```python
from build123d import *

# Parameters (mm, degrees)
SKETCH1_R           = 11.176
SKETCH1_R_2         = 1.5
BOSS_EXTRUDE1_DEPTH = 3.175


with BuildPart() as part:
    # Sketch1 → Boss-Extrude1 (new body)
    with BuildSketch(Plane.XY):
        with BuildLine():
            Line((-19.05, -19.05), (-19.05, 0))
            ThreePointArc((-19.05, 0), (0, 19.05), (19.05, 0))
            Line((19.05, 0), (19.05, -4.05))
            ThreePointArc((19.05, -4.05), (23.443398282, -14.656601718), (34.05, -19.05))
            Line((34.05, -19.05), (178.2, -19.05))
            ThreePointArc((178.2, -19.05), (188.806601718, -14.656601718), (193.2, -4.05))
            Line((193.2, -4.05), (193.2, 0))
            ThreePointArc((193.2, 0), (212.25, 19.05), (231.3, 0))
            Line((231.3, 0), (231.3, -19.05))
            Line((231.3, -19.05), (231.3, -79.925453532))
            Line((231.3, -79.925453532), (-19.05, -79.925453532))
            Line((-19.05, -79.925453532), (-19.05, -19.05))
        make_face()
        Circle(SKETCH1_R, mode=Mode.SUBTRACT)
        with Locations((212.25, 0)):
            Circle(SKETCH1_R, mode=Mode.SUBTRACT)
        with Locations((0, 13.9954)):
            Circle(SKETCH1_R_2, mode=Mode.SUBTRACT)
        with Locations((212.25, 13.9954)):
            Circle(SKETCH1_R_2, mode=Mode.SUBTRACT)
        with Locations((13.9954, 0)):
            Circle(SKETCH1_R_2, mode=Mode.SUBTRACT)
        with Locations((0, -13.9954)):
            Circle(SKETCH1_R_2, mode=Mode.SUBTRACT)
        with Locations((-13.9954, 0)):
            Circle(SKETCH1_R_2, mode=Mode.SUBTRACT)
        with Locations((198.2546, 0)):
            Circle(SKETCH1_R_2, mode=Mode.SUBTRACT)
        with Locations((212.25, -13.9954)):
            Circle(SKETCH1_R_2, mode=Mode.SUBTRACT)
        with Locations((226.2454, 0)):
            Circle(SKETCH1_R_2, mode=Mode.SUBTRACT)
    extrude(amount=BOSS_EXTRUDE1_DEPTH)


solid = part.part
```
Part model, mm, in its own coordinate system. A direction names the side the tool comes from. Give positions to 0.01 mm unless a question says otherwise; leave off trailing zeros. Write each loop counter-clockwise with the first axis right and the second up, starting at its lowest first coordinate (ties: lowest second). Pieces come first, ordered by that corner, then holes. Notation, with made-up numbers: (7.25, 26.5) -> (39.25, 26.5) arc R15 ccw to (39.25, 46.5) -> close; hole circle Ø10 at (26.5, -6). An arc over 180 degrees is marked (long way). Put each result on its own line as item: value. Start each with the question number.
Item 1: Cut at A-A (z = 1.4). State how many separate pieces and enclosed holes the cut face has, then the cut area to 3 significant figures.
Item 2: Wall check: L1, parallel to Y at x = 0, z = 1.2; L2, parallel to Y at x = 96, z = 1.85; L3, parallel to Y at x = 217.5, z = 1.65. Give the ranges that are in metal, low to high. Write a range as [from, to].
Item 3: Pin check, flat tips, straight feed: pin 1 Ø2.5 at (x, y) = (212.25, -14) entering from +Z; pin 2 Ø1 at (x, z) = (125.5, 2) entering from +Y. Stop position of each tip, or through.
Item 4: Which spindle directions (+Z, -Z, +X, -X, +Y, -Y) get a long thin tool onto all of the face, cutting with end or side? Do faces 3 (the face through (23.33, -14.54, 1.57)), 4 (the face through (108, -52, 3.175)). Say none if no direction does.
Item 5: Pull direction X, two halves, no side cores. Call faces 1 (the face through (-8.87, -6.8, 1.57)), 2 (the face through (108, -52, 0)): pulls with the +X half, pulls with the -X half, needs draft (parallel to the pull), parting line crosses it, or undercut.
Item 6: Cut at B-B (x = 138.5). List the corners of the cut face in (y, z) (3 decimals), then the cut area to 3 significant figures.
Answer list:
1. separate pieces: 1
1. enclosed holes: 10
1. area: 17,100 mm2
2. L1: y = [-79.93, -15.5], [-12.5, -11.18], [11.18, 12.5], [15.5, 19.05]
2. L2: y = [-79.93, -19.05]
2. L3: y = [-79.93, -9.87], [9.87, 18.31]
3. pin 1: passes through
3. pin 2: stops at y = -19.05
4. face 3: +Z, -Z, +Y
4. face 4: +Z, +X, -X, +Y, -Y
5. face 1: undercut
5. face 2: needs draft
6. outline: (-79.925, 0) -> (-19.05, 0) -> (-19.05, 3.175) -> (-79.925, 3.175) -> close
6. area: 193 mm2
